Geometry: final body of the model. Coordinates: model frame, mm. Round coordinates to 2 decimals unless told otherwise and drop trailing zeros. Order: outer loops, then holes, each group sorted by start corner. A loop starts at its lowest first (then second) coordinate and runs counter-clockwise, first axis right, second up. Notation, with made-up numbers: M -4,-32 L 1,-32 A20 ccw 1,-21 Z; hole C -8.75,4 d5. An arc over 180 degrees is marked long. Put each result on its own line as item: value. Start each with the question number.
1) Section A-A, the plane z = 21.5. Return loops of the section in (x, y) (3 decimals).
2) Material intervals for probe 1 along Y at (x, z) = (0.25, 22.5); probe 2 along X at (y, z) = (1.5, 10.5), sorted ascending. Write a range as [from, to].
3) First-contact query: P1, Ø1.5, axis at x = -1, z = 41.5, coming from the -Y side; P2, Ø1, axis at y = -0.5, z = 47, coming from the +X side (3 decimals); P3, Ø1.5, axis at y = -2.5, z = 61.5, coming from the +X side. Flat tips, straight axial feed; report the tip coordinate or a pass-through.
4) Section B-B, the plane y = 2.25. Return loops of the section in (x, z).
5) Section C-C, the plane x = 1. Return loops of the section in (y, z).
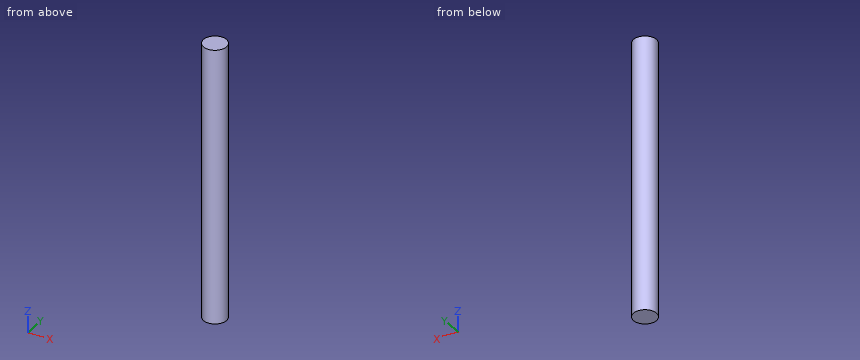
from build123d import *

# Parameters (mm, degrees)
F0_R     = 3.175
F1_DEPTH = 76.2
F2_DEPTH = 25.4
F3_DEPTH = 25.4


with BuildPart() as f1:
    # F0 (on Top) → F1 (new body)
    with BuildSketch(Plane.XY):
        Circle(F0_R)
    extrude(amount=F1_DEPTH)

    # F2 (cut): a face of the model
    f2_faces = [f1.faces().sort_by_distance(p)[0] for p in [
        (0, 0, 76.2),
    ]]
    extrude(f2_faces, amount=-F2_DEPTH, mode=Mode.SUBTRACT)

    # F3 (add): a face of the model
    f3_faces = [f1.faces().sort_by_distance(p)[0] for p in [
        (0, 0, 50.8),
    ]]
    extrude(f3_faces, amount=F3_DEPTH)


solid = f1.part
Result sheet:
1. outline: C 0,0 d6.35
2. probe 1: y = [-3.17, 3.17]
2. probe 2: x = [-2.8, 2.8]
3. P1: stops at y = -3.17
3. P2: stops at x = 3.175
3. P3: stops at x = 2.65
4. outline: M -2.24,0 L 2.24,0 L 2.24,76.2 L -2.24,76.2 Z
5. outline: M -3.01,0 L 3.01,0 L 3.01,76.2 L -3.01,76.2 Z
